Part print with two shaded views. Sizes in mm from the minimum x, y, z corner. A direction names the side the tool comes from. Round coordinates to 2 decimals unless told otherwise and drop trailing zeros. Loops run counter-clockwise (first coordinate to the right, second up) from the corner with the lowest first, then second, coordinate; pieces in that order, holes last.
(1) Cut at D-D on x = 14.5. List the corners of the cut face in (y, z).
(2) Mould opens along Y. For the marked faces 4, 5 and 6 say: +Y half, -Y half, draft (parallel to the pull), parting line (faces both ways), or undercut.
(3) Flat gauge pins, fed straight in: pin 1 (3 mm diameter, centred on y = 2, z = 1.5, fed in from +X); pin 2 (8 mm diameter, centred on x = 14, y = 9.5, fed in from +Z); pin 3 (3 mm diameter, centred on x = 2, z = 1.5, fed in from +Y). Where does each tip first touch, or does it go through?
(4) Tool access for the marked faces 1, 2 and 3: list every direction of +Z, -Z, +X, -X, +Y, -Y with a clear straight run to the whole face (end or side of a thin tool).
(5) Probe probe 1 along Y at (x, z) = (8, 4.95) (1 decimal); probe 2 along Y at (x, z) = (8, 1.85); probe 3 along Z at (x, y) = (6.5, 14.5). List the from-to ranges inside material, lowest first.
(6) Cut at C-C on z = 2.85. List the corners of the cut face in (x, y).
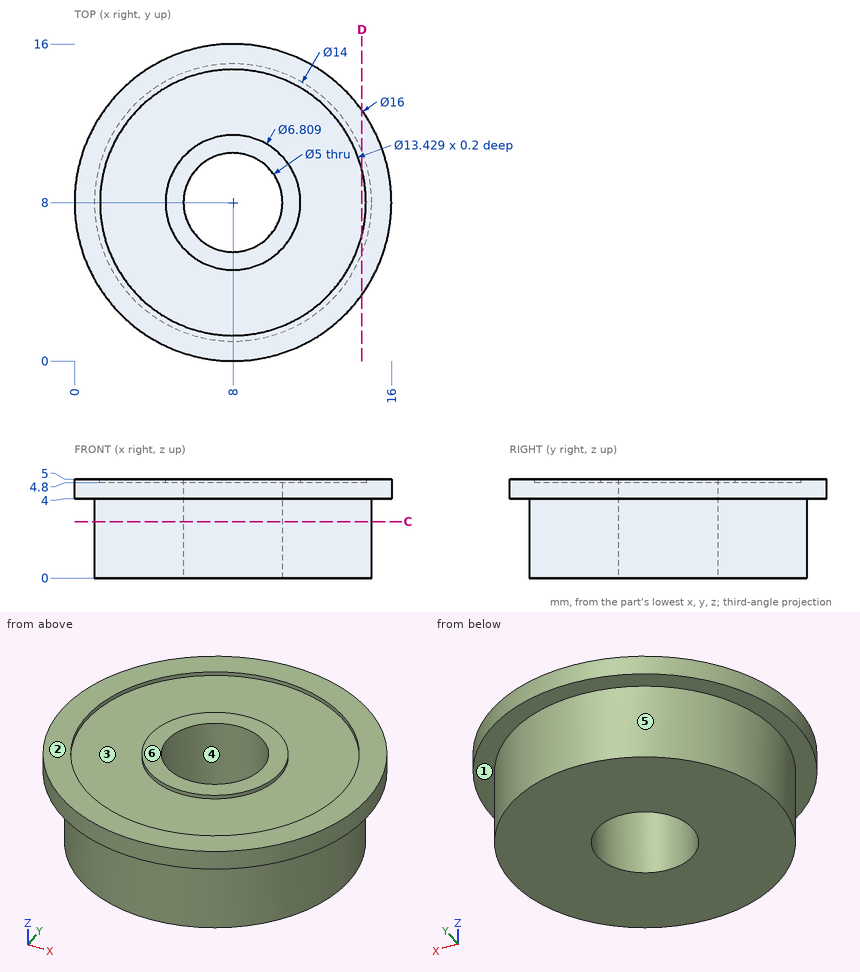
Final values:
1. outline: (3.34, 4) - (5.4, 4) - (5.4, 0) - (10.6, 0) - (10.6, 4) - (12.66, 4) - (12.66, 5) - (9.68, 5) - (9.68, 4.8) - (6.32, 4.8) - (6.32, 5) - (3.34, 5) - close
2. face 4: undercut
2. face 5: parting line
2. face 6: draft
3. pin 1: stops at x = 13.36
3. pin 2: stops at z = 5
3. pin 3: stops at y = 13.36
4. face 1: -Z
4. face 2: +Z, +X, -X, +Y, -Y
4. face 3: +Z
5. probe 1: y = 0 to 1.3, 4.6 to 5.5, 10.5 to 11.4, 14.7 to 16
5. probe 2: y = 1 to 5.5, 10.5 to 15
5. probe 3: z = 0 to 4.8
6. outline: circle Ø14 at (8, 8); hole circle Ø5 at (8, 8)
